Input: part model. Units: mm. Frame: model coordinates. Face numbers are marked on the shaded views. Coordinates: 2 decimals unless noted, no trailing zeros. Write each loop counter-clockwise with the first axis right and the second up, starting at its lowest first coordinate (ties: lowest second). Pieces come first, ordered by that corner, then holes. Notation, with made-up numbers: (39.5, 44) - (48.5, 44) arc R23 cw to (48.5, 66) - close; hole circle Ø2 at (79.5, -35). An arc over 180 degrees is marked (long way). Use CSV: the item, a comma, the result in double quotes.
```python
from build123d import *

# Parameters (mm, degrees)
SKETCH19_W               = 895
SKETCH19_H               = 180
SKETCH19_W_2             = 865
SKETCH19_H_2             = 150
BOSS_EXTRUDE2_DEPTH      = 48
SKETCH22_W               = 895
SKETCH22_H               = 180
BOSS_EXTRUDE3_DEPTH      = 10
BOSS_EXTRUDE4_DEPTH      = 56
BOSS_EXTRUDE4_DEPTH_BACK = 10
SKETCH23_W               = 1500
SKETCH23_H               = 500
SKETCH23_W_2             = 895
SKETCH23_H_2             = 180
CUT_EXTRUDE6_START       = 48
SKETCH26_R               = 1.65
CUT_EXTRUDE6_DEPTH       = 20
LPATTERN1_COUNT          = 5
LPATTERN1_PITCH          = 220
SKETCH28_R               = 2.3
SKETCH28_R_2             = 57.7
CUT_EXTRUDE7_DEPTH       = 793.55031386
LPATTERN2_COUNT          = 2
LPATTERN2_PITCH          = 350
LPATTERN2_COL_COUNT      = 2
LPATTERN2_COL_PITCH      = 350
CUT_EXTRUDE8_START       = 48
SKETCH27_R               = 1.65
CUT_EXTRUDE8_DEPTH       = 20
CUT_EXTRUDE9_START       = -56
CUT_EXTRUDE9_DEPTH       = 2
CUT_EXTRUDE10_START      = 56
CUT_EXTRUDE10_DEPTH      = 2
CUT_EXTRUDE11_DEPTH      = 793.55031386
CUT_EXTRUDE11_DEPTH_BACK = 793.55031386
SKETCH33_R               = 2.35
CUT_EXTRUDE12_DEPTH      = 793.55031386
CUT_EXTRUDE12_DEPTH_BACK = 793.55031386
SKETCH34_W               = 190.830831748
SKETCH34_H               = 540.530008981
SKETCH29_W               = 150
SKETCH29_H               = 100
BOSS_EXTRUDE5_DEPTH      = 50
CUT_EXTRUDE13_START      = 56
SKETCH35_W               = 15
SKETCH35_H               = 100
CUT_EXTRUDE13_DEPTH      = 15
SKETCH36_R               = 1.3
CUT_EXTRUDE14_DEPTH      = 10
SKETCH37_R               = 2.25
CUT_EXTRUDE15_DEPTH      = 10


with BuildPart() as part:
    # Sketch19 → Boss-Extrude2 (new body)
    with BuildSketch(Plane(origin=(0, 0, 0), x_dir=(1, 0, 0), z_dir=(0, 1, 0))):
        Rectangle(SKETCH19_W, SKETCH19_H)
        Rectangle(SKETCH19_W_2, SKETCH19_H_2, mode=Mode.SUBTRACT)
    extrude(amount=BOSS_EXTRUDE2_DEPTH)

    # Sketch22 → Boss-Extrude3 (add)
    with BuildSketch(Plane(origin=(0, 0, 0), x_dir=(1, 0, 0), z_dir=(0, 1, 0))):
        Rectangle(SKETCH22_W, SKETCH22_H)
    extrude(amount=-BOSS_EXTRUDE3_DEPTH)

    # Sketch23 → Boss-Extrude4 (add, two sides: drawn at the far end of the back side and taken through both)
    with BuildSketch(Plane(origin=(0, 0, 0), x_dir=(1, 0, 0), z_dir=(0, 1, 0)).offset(-BOSS_EXTRUDE4_DEPTH_BACK)):
        Rectangle(SKETCH23_W, SKETCH23_H)
        Rectangle(SKETCH23_W_2, SKETCH23_H_2, mode=Mode.SUBTRACT)
    extrude(amount=BOSS_EXTRUDE4_DEPTH + BOSS_EXTRUDE4_DEPTH_BACK)

    # Sketch26 → Cut-Extrude6 (cut)
    with BuildSketch(Plane(origin=(0, 0, 0), x_dir=(1, 0, 0), z_dir=(0, 1, 0)).offset(CUT_EXTRUDE6_START)):
        with Locations(Location((-440, -82.5, 0), (0, 0, 90))):
            Circle(SKETCH26_R)
        with Locations(Location((-440, 82.5, 0), (0, 0, 90))):
            Circle(SKETCH26_R)
    cut_extrude6 = extrude(amount=-CUT_EXTRUDE6_DEPTH, mode=Mode.SUBTRACT)

    # LPattern1: Cut-Extrude6 ×5
    with Locations(*[(i * LPATTERN1_PITCH, 0, 0) for i in range(1, LPATTERN1_COUNT)]):
        add(cut_extrude6, mode=Mode.SUBTRACT)

    # Sketch28 → Cut-Extrude7 (cut, symmetric)
    with BuildSketch(Plane(origin=(0, 0, 0), x_dir=(1, 0, 0), z_dir=(0, 1, 0))):
        with Locations(Location((-52.5, 52.5, 0), (0, 0, 270))):
            Circle(SKETCH28_R)
        with Locations(Location((52.5, 52.5, 0), (0, 0, 270))):
            Circle(SKETCH28_R)
        with Locations(Location((52.5, -52.5, 0), (0, 0, 270))):
            Circle(SKETCH28_R)
        with Locations(Location((-52.5, -52.5, 0), (0, 0, 270))):
            Circle(SKETCH28_R)
        with Locations(Location((0, 0, 0), (0, 0, 270))):
            Circle(SKETCH28_R_2)
    cut_extrude7 = extrude(amount=CUT_EXTRUDE7_DEPTH, both=True, mode=Mode.SUBTRACT)

    # LPattern2: Cut-Extrude7 ×2
    with Locations(*[(-i * LPATTERN2_PITCH, 0, 0) for i in range(1, LPATTERN2_COUNT)]):
        add(cut_extrude7, mode=Mode.SUBTRACT)

    # LPattern2 col: Cut-Extrude7 ×2
    with Locations(*[(i * LPATTERN2_COL_PITCH, 0, 0) for i in range(1, LPATTERN2_COL_COUNT)]):
        add(cut_extrude7, mode=Mode.SUBTRACT)

    # Sketch27 → Cut-Extrude8 (cut)
    with BuildSketch(Plane(origin=(0, 0, 0), x_dir=(1, 0, 0), z_dir=(0, 1, 0)).offset(CUT_EXTRUDE8_START)):
        with Locations(Location((-440, 27.5, 0), (0, 0, 90))):
            Circle(SKETCH27_R)
        with Locations(Location((-440, -35, 0), (0, 0, 90))):
            Circle(SKETCH27_R)
        with Locations(Location((440, -35, 0), (0, 0, 90))):
            Circle(SKETCH27_R)
        with Locations(Location((440, 27.5, 0), (0, 0, 90))):
            Circle(SKETCH27_R)
    extrude(amount=-CUT_EXTRUDE8_DEPTH, mode=Mode.SUBTRACT)

    # Sketch30 → Cut-Extrude9 (cut)
    with BuildSketch(Plane.XZ.offset(CUT_EXTRUDE9_START)):
        with BuildLine():
            Line((571.5, -147.92), (714.5, -147.92))
            ThreePointArc((714.5, -147.92), (715.207106781, -147.627106781), (715.5, -146.92))
            Line((715.5, -146.92), (715.5, -89.92))
            ThreePointArc((715.5, -89.92), (715.207106781, -89.212893219), (714.5, -88.92))
            Line((714.5, -88.92), (571.5, -88.92))
            ThreePointArc((571.5, -88.92), (567.964466094, -90.384466094), (566.5, -93.92))
            Line((566.5, -93.92), (566.5, -142.92))
            ThreePointArc((566.5, -142.92), (567.964466094, -146.455533906), (571.5, -147.92))
        make_face()
    cut_extrude9 = extrude(amount=CUT_EXTRUDE9_DEPTH, mode=Mode.SUBTRACT)

    # Mirror1: Cut-Extrude9 across plane
    add(cut_extrude9.mirror(Plane.XY), mode=Mode.SUBTRACT)

    # Sketch32 → Cut-Extrude10 (cut)
    with BuildSketch(Plane(origin=(0, 0, 0), x_dir=(1, 0, 0), z_dir=(0, 1, 0)).offset(CUT_EXTRUDE10_START)):
        with BuildLine():
            Line((-591.5, 147.92), (-571.5, 147.92))
            ThreePointArc((-571.5, 147.92), (-567.964466094, 146.455533906), (-566.5, 142.92))
            Line((-566.5, 142.92), (-566.5, 93.92))
            ThreePointArc((-566.5, 93.92), (-567.964466094, 90.384466094), (-571.5, 88.92))
            Line((-571.5, 88.92), (-591.5, 88.92))
            ThreePointArc((-591.5, 88.92), (-595.035533906, 90.384466094), (-596.5, 93.92))
            Line((-596.5, 93.92), (-596.5, 142.92))
            ThreePointArc((-596.5, 142.92), (-595.035533906, 146.455533906), (-591.5, 147.92))
        make_face()
    cut_extrude10 = extrude(amount=-CUT_EXTRUDE10_DEPTH, mode=Mode.SUBTRACT)

    # Mirror2: Cut-Extrude10 across plane
    add(cut_extrude10.mirror(Plane.XY), mode=Mode.SUBTRACT)

    # Sketch33 → Cut-Extrude11 (cut, two sides: drawn at the far end of the back side and taken through both)
    with BuildSketch(Plane(origin=(0, 0, 0), x_dir=(1, 0, 0), z_dir=(0, 1, 0)).offset(-CUT_EXTRUDE11_DEPTH_BACK)):
        with Locations(Location((-581.5, 108.58, 0), (0, 0, 270))):
            Circle(SKETCH33_R)
        with Locations(Location((-581.5, -108.59, 0), (0, 0, 270))):
            Circle(SKETCH33_R)
        with Locations(Location((-581.5, 128.25, 0), (0, 0, 270))):
            Circle(SKETCH33_R)
        with Locations(Location((-581.5, -128.26, 0), (0, 0, 270))):
            Circle(SKETCH33_R)
        with Locations(Location((616.17, -118.42, 0), (0, 0, 270))):
            Circle(SKETCH33_R)
        with Locations(Location((665.84, -118.42, 0), (0, 0, 270))):
            Circle(SKETCH33_R)
        with Locations(Location((616.17, 118.42, 0), (0, 0, 270))):
            Circle(SKETCH33_R)
        with Locations(Location((665.84, 118.42, 0), (0, 0, 270))):
            Circle(SKETCH33_R)
    extrude(amount=CUT_EXTRUDE11_DEPTH + CUT_EXTRUDE11_DEPTH_BACK, mode=Mode.SUBTRACT)

    # Sketch34 → Cut-Extrude12 (cut, two sides: drawn at the far end of the back side and taken through both)
    with BuildSketch(Plane(origin=(0, 0, 0), x_dir=(1, 0, 0), z_dir=(0, 1, 0)).offset(-CUT_EXTRUDE12_DEPTH_BACK)):
        with Locations((-726.415415874, 20.265004491)):
            Rectangle(SKETCH34_W, SKETCH34_H)
    extrude(amount=CUT_EXTRUDE12_DEPTH + CUT_EXTRUDE12_DEPTH_BACK, mode=Mode.SUBTRACT)

    # Sketch29 → Boss-Extrude5 (add)
    with BuildSketch(Plane(origin=(0, 0, 0), x_dir=(1, 0, 0), z_dir=(0, 1, 0))):
        with Locations((-556, -200)):
            Rectangle(SKETCH29_W, SKETCH29_H)
        with Locations((-556, 200)):
            Rectangle(SKETCH29_W, SKETCH29_H)
        with Locations((675, -200)):
            Rectangle(SKETCH29_W, SKETCH29_H)
        with Locations((675, 200)):
            Rectangle(SKETCH29_W, SKETCH29_H)
    extrude(amount=-BOSS_EXTRUDE5_DEPTH)

    # Sketch35 → Cut-Extrude13 (cut)
    with BuildSketch(Plane(origin=(0, 0, 0), x_dir=(1, 0, 0), z_dir=(0, 1, 0)).offset(CUT_EXTRUDE13_START)):
        with Locations((-440, -200)):
            Rectangle(SKETCH35_W, SKETCH35_H)
    extrude(amount=-CUT_EXTRUDE13_DEPTH, mode=Mode.SUBTRACT)

    # Sketch36 → Cut-Extrude14 (cut)
    with BuildSketch(Plane(origin=(0, 56, 0), x_dir=(-1, 0, 0), z_dir=(0, 1, 0))):
        with Locations(Location((-683.996319, -14.497340105, 0), (0, 0, 90))):
            Circle(SKETCH36_R)
        with Locations(Location((-683.996319, -63.497340105, 0), (0, 0, 90))):
            Circle(SKETCH36_R)
        with Locations(Location((-625.996319, -63.497340105, 0), (0, 0, 90))):
            Circle(SKETCH36_R)
        with Locations(Location((-625.996319, -14.497340105, 0), (0, 0, 90))):
            Circle(SKETCH36_R)
    extrude(amount=-CUT_EXTRUDE14_DEPTH, mode=Mode.SUBTRACT)

    # Sketch37 → Cut-Extrude15 (cut)
    with BuildSketch(Plane(origin=(0, 56, 0), x_dir=(1, 0, 0), z_dir=(0, 1, 0))):
        with Locations(Location((717.160651903, -205, 0), (0, 0, 270))):
            Circle(SKETCH37_R)
        with Locations(Location((629.160651903, -205, 0), (0, 0, 270))):
            Circle(SKETCH37_R)
        with Locations(Location((591.138632586, -205, 0), (0, 0, 270))):
            Circle(SKETCH37_R)
        with Locations(Location((503.138632586, -205, 0), (0, 0, 270))):
            Circle(SKETCH37_R)
        with Locations(Location((717.160651903, 205, 0), (0, 0, 270))):
            Circle(SKETCH37_R)
        with Locations(Location((629.160651903, 205, 0), (0, 0, 270))):
            Circle(SKETCH37_R)
    extrude(amount=-CUT_EXTRUDE15_DEPTH, mode=Mode.SUBTRACT)


solid = part.part
```
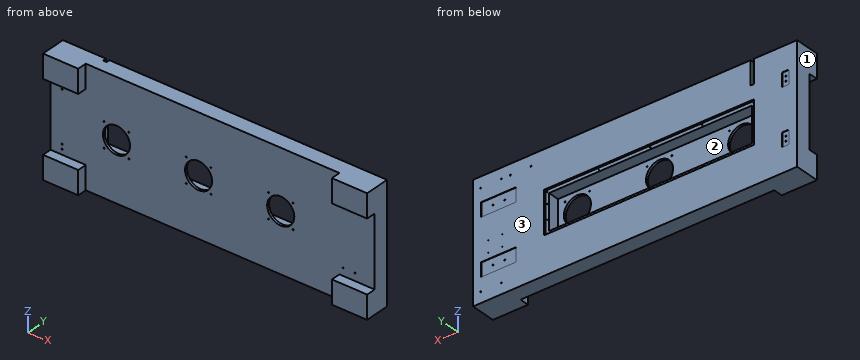
(1) Cut plane C-C on x = -87. Return loops of the section in (y, z).
Check values:
outline,"(-10, -250) - (56, -250) - (56, -90) - (48, -90) - (48, -75) - (0, -75) - (0, 75) - (48, 75) - (48, 90) - (56, 90) - (56, 250) - (-10, 250) - close"
(2) Draft query along X for the marked faces 1, 2 and 3. Return one class per face: pulls with the +X half, pulls with the -X half, needs draft (parallel to the pull), parting line crosses it, or undercut.
Check values:
face 1,"pulls with the -X half"
face 2,"undercut"
face 3,"needs draft"
(3) Cut plane A-A on z = 0. Return loops of the section in (x, y).
Check values:
outline,"(-631, -10) - (-407.7, -10) - (-407.7, 0) - (-432.5, 0) - (-432.5, 48) - (-447.5, 48) - (-447.5, 56) - (-631, 56) - close; (-292.3, -10) - (-57.7, -10) - (-57.7, 0) - (-292.3, 0) - close; (57.7, -10) - (292.3, -10) - (292.3, 0) - (57.7, 0) - close; (407.7, -10) - (750, -10) - (750, 56) - (447.5, 56) - (447.5, 48) - (432.5, 48) - (432.5, 0) - (407.7, 0) - close"
(4) Ray query, probe 1 along Z at (x, y) = (-581.5, 22); probe 2 along X at (y, z) = (35, -82.5); probe 3 along Z at (x, y) = (-440, 35). Return the intervals inside material, ascending. Write a range as from..to.
Check values:
probe 1,"-250..-130.6, -125.9..-110.93, -106.23..106.24, 110.94..125.91, 130.61..250"
probe 2,"-631..-441.65, -438.35..-221.65, -218.35..-1.65, 1.65..218.35, 221.65..438.35, 441.65..750"
probe 3,"-250..-84.15, -80.85..-29.15, -25.85..33.35, 36.65..80.85, 84.15..250"
(5) Pin query (flat end, axial travel): pin 1 Ø3 at (x, z) = (440, -82.5) entering from +Y; pin 2 Ø3 at (x, z) = (-250.5, -23) entering from -Y; pin 3 Ø1 at (x, z) = (-285.5, -78) entering from +Y. Return the tip coordinate at first contact, or that it passes through.
Check values:
pin 1,"y = 28"
pin 2,"y = -10"
pin 3,"y = 48"
(6) Cut plane B-B on y = -25. Return loops of the section in (x, z).
Check values:
outline,"(-631, -250) - (-481, -250) - (-481, -150) - (-631, -150) - close; (-631, 150) - (-481, 150) - (-481, 250) - (-631, 250) - close; (600, -250) - (750, -250) - (750, -150) - (600, -150) - close; (600, 150) - (750, 150) - (750, 250) - (600, 250) - close"
(7) Cut plane D-D on z = 182. Return loops of the section in (x, y).
Check values:
outline,"(-631, -50) - (-481, -50) - (-481, -10) - (600, -10) - (600, -50) - (750, -50) - (750, 56) - (-432.5, 56) - (-432.5, 41) - (-447.5, 41) - (-447.5, 56) - (-631, 56) - close"
